Design review of the part built by this model. Coordinates are the model's own, in mm. A direction names the side the tool comes from. Coordinates: 2 decimals unless noted, no trailing zeros. Write each loop counter-clockwise with the first axis right and the second up, starting at its lowest first coordinate (ties: lowest second). Pieces come first, ordered by that corner, then holes. Notation, with made-up numbers: (-12.5, -8) -> (24.5, -8) arc R28 cw to (24.5, 14) -> close; hole circle Ø3 at (44, 75). An arc over 180 degrees is marked (long way). Answer in a Markdown table with one row per item. Add a question column.
Item 1: Take a section at A-A, the plane y = 515. Write out the cut boundary in (x, z).
Item 2: Take a section at C-C, the plane y = 101. Write out the cut boundary in (x, z), and give its area (3 significant figures).
Item 3: To check wall thickness, follow line 1 (Y direction, x = 214, z = 81.75); line 2 (Y direction, x = 217, z = 81); line 3 (X direction, y = 515, z = 60). State the ranges of each line that lie inside material, in increasing order.
Item 4: Clearance check with flat-ended pins moving along their axes: P1, Ø4, axis at y = 591, z = 81, coming from the -X side; P2, Ø19, axis at x = 226, y = 101, coming from the -Z side; P3, Ø5, axis at x = 236.5, z = 63.5, coming from the -Y side; P4, Ø11, axis at x = 226, y = 515, coming from the +Z side. State where each tip first meets the part, or that it passes through.
Item 5: For faces 5 (the face through (218.242, 504.882, 42.887)), 6 (the face through (226, 616, 76)), 7 (the face through (210, 312, 64)), 8 (the face through (226, 595, 70.5)), 9 (the face through (226, 21, 70.5)), list the 3-axis set-ups (+Z, -Z, +X, -X, +Y, -Y) from which the entire face can be reached by the end or side of a thin tool; tool diameter is ignored.
Item 6: Draft analysis for pull direction Y (two halves, no side actions). For faces 1 (the face through (226, 486, 24)), 2 (the face through (225.78, 3.61, 89.58)), 3 (the face through (230, 96, 42)), 4 (the face through (220.5, 512, 43.8)), state which applies: released by +Y, released by -Y, zero draft, split by the parting line, or undercut.
Item 7: Take a section at B-B, the plane x = 226. Write out the cut boundary in (y, z).
from build123d import *

# Parameters (mm, degrees)
PAD027_DEPTH            = 32
POCKET047_DEPTH         = 32
POCKET048_DEPTH         = 32
SKETCH079_R             = 4
POCKET049_DEPTH         = 10
SKETCH080_R             = 6
POCKET050_DEPTH         = 51
SKETCH081_R             = 12.75
POCKET051_DEPTH         = 1.8
BODY026_ROLL_ANGLE      = 90
BODY026_PLACEMENT_ANGLE = 90


with BuildPart() as part:
    # Sketch076 → Pad027 (new body)
    with BuildSketch(Plane.XY):
        with BuildLine():
            Line((-296, 75), (296, 75))
            ThreePointArc((308, 63), (304.485281, 71.485281), (296, 75))
            Line((308, 63), (308, 0))
            Line((308, 0), (-308, 0))
            Line((-308, 0), (-308, 63))
            ThreePointArc((-296, 75), (-304.485281, 71.485281), (-308, 63))
        make_face()
    extrude(amount=PAD027_DEPTH)

    # Sketch077 (on Face8 of Pad027) → Pocket047 (cut)
    with BuildSketch(Plane.XY.offset(32)):
        with BuildLine():
            Line((-308, 24), (-190, 24))
            ThreePointArc((-178, 12), (-181.514719, 20.485281), (-190, 24))
            Line((-178, 12), (-178, 0))
            Line((-178, 0), (-308, 0))
            Line((-308, 0), (-308, 24))
        make_face()
    pocket047 = extrude(amount=-POCKET047_DEPTH, mode=Mode.SUBTRACT)

    # Mirrored018: Pocket047 across Sketch077 V_Axis
    add(pocket047.mirror(Plane(origin=(0, 0, 32), x_dir=(0, 0, 1), z_dir=(1, 0, 0))), mode=Mode.SUBTRACT)

    # Sketch078 (on Face4 of Mirrored018) → Pocket048 (cut)
    with BuildSketch(Plane.XY.offset(32)):
        with BuildLine():
            ThreePointArc((-264.5, -28.5), (-224, 12), (-264.5, 52.5))
            Line((-345.5, 52.5), (-264.5, 52.5))
            Line((-345.5, -28.5), (-345.5, 52.5))
            Line((-264.5, -28.5), (-345.5, -28.5))
        make_face()
    pocket048 = extrude(amount=-POCKET048_DEPTH, mode=Mode.SUBTRACT)

    # Mirrored019: Pocket048 across Sketch078 V_Axis
    add(pocket048.mirror(Plane(origin=(0, 0, 32), x_dir=(0, 0, 1), z_dir=(1, 0, 0))), mode=Mode.SUBTRACT)

    # Sketch079 (on Face2 of Mirrored019) → Pocket049 (cut)
    with BuildSketch(Plane(origin=(0, 0, 0), x_dir=(1, 0, 0), z_dir=(0, 0, -1))):
        with Locations((-284, -63.75)):
            Circle(SKETCH079_R)
        with Locations((-102.666667, -25)):
            Circle(SKETCH079_R)
        with Locations((0, -25)):
            Circle(SKETCH079_R)
        with Locations((102.666667, -25)):
            Circle(SKETCH079_R)
        with Locations((284, -63.75)):
            Circle(SKETCH079_R)
    extrude(amount=-POCKET049_DEPTH, mode=Mode.SUBTRACT)

    # Sketch080 (on Face9 of Pocket049) → Pocket050 (cut)
    with BuildSketch(Plane.XZ.offset(-24)):
        with Locations((207, 16)):
            Circle(SKETCH080_R)
    pocket050 = extrude(amount=-POCKET050_DEPTH, mode=Mode.SUBTRACT)

    # Sketch081 (on Face9 of Pocket050) → Pocket051 (cut)
    with BuildSketch(Plane.XZ.offset(-24)):
        with Locations((207, 16)):
            Circle(SKETCH081_R)
    extrude(amount=-POCKET051_DEPTH, mode=Mode.SUBTRACT)

    # Mirrored020: Pocket050 across Sketch080 V_Axis
    add(pocket050.mirror(Plane(origin=(0, 24, 0), x_dir=(0, -1, 0), z_dir=(1, 0, 0))), mode=Mode.SUBTRACT)


with BuildPart() as part_1:
    # Body026 roll: moved
    add(part.part.rotate(Axis((0, 0, 0), (1, 0, 0)), BODY026_ROLL_ANGLE))


with BuildPart() as part_2:
    # Body026 placement: moved
    add(part_1.part.moved(Location((210, 308, 18))).rotate(Axis((210, 308, 18), (0, 0, 1)), BODY026_PLACEMENT_ANGLE))


solid = part_2.part
Answers:
| question | item | result |
|---|---|---|
| 1 | outline | (210, 42) -> (213.25, 42) -> (213.25, 43.8) -> (220, 43.8) -> (220, 93) -> (210, 93) -> close; (232, 43.8) -> (238.75, 43.8) -> (238.75, 42) -> (242, 42) -> (242, 93) -> (232, 93) -> close |
| 2 | outline | (210, 42) -> (220, 42) -> (220, 93) -> (210, 93) -> close; (232, 42) -> (242, 42) -> (242, 93) -> (232, 93) -> close |
| 2 | area | 1,020 mm^2 |
| 3 | line 1 | y = 0.02 to 20, 28 to 588, 596 to 615.98 |
| 3 | line 2 | y = 0 to 20.07, 27.93 to 588.07, 595.93 to 616 |
| 3 | line 3 | x = 210 to 220, 232 to 242 |
| 4 | P1 | stops at x = 220 |
| 4 | P2 | stops at z = 42 |
| 4 | P3 | stops at y = 62.05 |
| 4 | P4 | passes through |
| 5 | face 5 | -Z |
| 5 | face 6 | +Z, -Z, +X, -X, +Y |
| 5 | face 7 | +Z, -Z, -X, +Y, -Y |
| 5 | face 8 | -Z, +X, -X, +Y |
| 5 | face 9 | -Z, +X, -X, -Y |
| 6 | face 1 | released by +Y |
| 6 | face 2 | released by -Y |
| 6 | face 3 | zero draft |
| 6 | face 4 | undercut |
| 7 | outline | (0, 70.5) -> (43.5, 70.5) arc R40.5 cw to (82.18, 42) -> (95, 42) -> (95, 93) -> (12, 93) arc R12 ccw to (0, 81) -> close; (107, 42) -> (118, 42) arc R12 cw to (130, 30) -> (130, 18) -> (486, 18) -> (486, 30) arc R12 cw to (498, 42) -> (502.25, 42) -> (502.25, 43.8) -> (509, 43.8) -> (509, 93) -> (107, 93) -> close; (521, 43.8) -> (527.75, 43.8) -> (527.75, 42) -> (533.82, 42) arc R40.5 cw to (572.5, 70.5) -> (616, 70.5) -> (616, 81) arc R12 ccw to (604, 93) -> (521, 93) -> close |
